The model under review builds one solid part; all positions refer to its coordinate system, in mm. Give positions to 0.01 mm unless a question says otherwise; leave off trailing zeros. Write each question's results on one line, items separated by ' | '. Start each with the question number.
from build123d import *

# Parameters (mm, degrees)
SKETCH_1_W             = 320
SKETCH_1_H             = 5
EXTRUDE_1_DEPTH        = 2
SKETCH_2_R             = 1.5
CUT_EXTRUDE_1_DEPTH    = 321.045309292
PATTERN_LINEAR_1_COUNT = 35
PATTERN_LINEAR_1_PITCH = 5
PATTERN_LINEAR_2_COUNT = 35
PATTERN_LINEAR_2_PITCH = 5


with BuildPart() as part:
    # 草图1 → 凸台-拉伸1 (new body)
    with BuildSketch(Plane.XY):
        with Locations((160, -2.5)):
            Rectangle(SKETCH_1_W, SKETCH_1_H)
    extrude(amount=EXTRUDE_1_DEPTH)

    # 草图2 → 切除-拉伸1 (cut, through all)
    with BuildSketch(Plane.XY.offset(2)):
        with Locations((160, -2.5)):
            Circle(SKETCH_2_R)
    cut_extrude_1 = extrude(amount=-CUT_EXTRUDE_1_DEPTH, mode=Mode.SUBTRACT)

    # 阵列(线性)1: 切除-拉伸1 ×35
    with Locations(*[(i * PATTERN_LINEAR_1_PITCH, 0, 0) for i in range(1, PATTERN_LINEAR_1_COUNT)]):
        add(cut_extrude_1, mode=Mode.SUBTRACT)

    # 阵列(线性)2: 切除-拉伸1 ×35
    with Locations(*[(-i * PATTERN_LINEAR_2_PITCH, 0, 0) for i in range(1, PATTERN_LINEAR_2_COUNT)]):
        add(cut_extrude_1, mode=Mode.SUBTRACT)


solid = part.part
(1) Draft analysis for pull direction Z (two halves, no side actions). For faces 1 (the flat face through (158, -2, 0)), 2 (the flat face through (158, -2, 2)), state which applies: pulls with the +Z half, pulls with the -Z half, needs draft (parallel to the pull), parting line crosses it, or undercut.
(2) Clearance check with a flat-ended pin moving along its axis: P1, Ø2.5, axis at x = 75, y = -2.5, coming from the +Z side. State where the tip first meets the part, or that it passes through.
(3) Add section A-A (z = 0.7). Give the number of separate pieces and of enclosed holes in the cut face, then the cut area to 3 significant figures.
(4) Wall thickness on L1, parallel to Y at x = 145, z = 1.5; L2, parallel to Y at x = 290.5, z = 0.75: over which ranges is each line inside the solid? List them lowest first.
Calculated:
1) face 1: pulls with the -Z half | face 2: pulls with the +Z half
2) P1: passes through
3) separate pieces: 1 | enclosed holes: 63 | area: 1,150 mm²
4) L1: y = -5 to -4, -1 to 0 | L2: y = -5 to -3.91, -1.09 to 0
